Input: dimensioned drawing with shaded views. Units: mm. Origin: part minimum x, y, z. Round coordinates to 2 decimals unless told otherwise and drop trailing zeros. Loops run counter-clockwise (first coordinate to the right, second up) from the corner with the lowest first, then second, coordinate; pieces in that order, holes last.
Item 1: Section query A-A on x = 121.5. Return loops of the section in (y, z), then the cut area to 3 significant figures.
Item 2: Section query D-D on y = 118. Return loops of the section in (x, z).
Item 3: Ray query, L1, parallel to Y at x = 40.5, z = 3.9 (1 decimal); L2, parallel to Y at x = 37, z = 0.4 (1 decimal); L3, parallel to Y at x = 121.5, z = 2.4. Return the intervals inside material, ascending.
Item 4: Section query B-B on y = 67.5. Return loops of the section in (x, z), then the cut area to 3 significant figures.
Item 5: First-contact query: P1, Ø11, axis at x = 40.5, y = 114.27, coming from the -Z side; P2, Ø2, axis at x = 110.5, z = 1, coming from the +Y side. Flat tips, straight axial feed; report the tip coordinate or a pass-through.
Item 6: Section query C-C on x = 40.5. Return loops of the section in (y, z) (1 decimal).
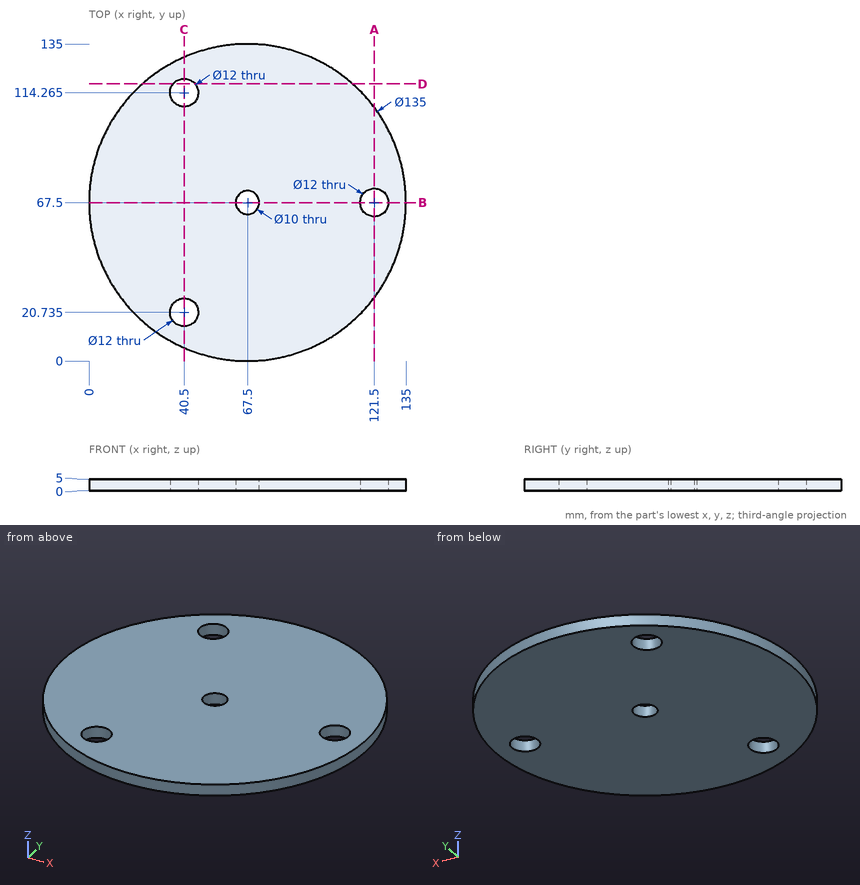
Data:
1. outline: (27, 0) - (61.5, 0) - (61.5, 5) - (27, 5) - close; (73.5, 0) - (108, 0) - (108, 5) - (73.5, 5) - close
1. area: 345 mm2
2. outline: (22.71, 0) - (35.8, 0) - (35.8, 5) - (22.71, 5) - close; (45.2, 0) - (112.29, 0) - (112.29, 5) - (45.2, 5) - close
3. L1: y = 5.6 to 14.7, 26.7 to 108.3, 120.3 to 129.4
3. L2: y = 7.3 to 15.9, 25.6 to 109.4, 119.1 to 127.7
3. L3: y = 27 to 61.5, 73.5 to 108
4. outline: (0, 0) - (62.5, 0) - (62.5, 5) - (0, 5) - close; (72.5, 0) - (115.5, 0) - (115.5, 5) - (72.5, 5) - close; (127.5, 0) - (135, 0) - (135, 5) - (127.5, 5) - close
4. area: 565 mm2
5. P1: passes through
5. P2: stops at y = 120.34
6. outline: (5.6, 0) - (14.7, 0) - (14.7, 5) - (5.6, 5) - close; (26.7, 0) - (108.3, 0) - (108.3, 5) - (26.7, 5) - close; (120.3, 0) - (129.4, 0) - (129.4, 5) - (120.3, 5) - close
